The listing builds one solid part. Answer for the finished solid, in the listing's coordinates (mm). Give positions to 0.01 mm unless a question says otherwise; leave off trailing zeros. Order: outer loops, then holes, each group sorted by start corner. A loop starts at its lowest first (then second) coordinate and runs counter-clockwise, first axis right, second up. Notation, with made-up numbers: (21.5, 89.5) - (62.5, 89.5) arc R25 ccw to (62.5, 106.5) - close; hole circle Ø3 at (-22, 60.5). An arc over 180 degrees is marked (long way). Answer in a Markdown table with one row per item. Add a question column.
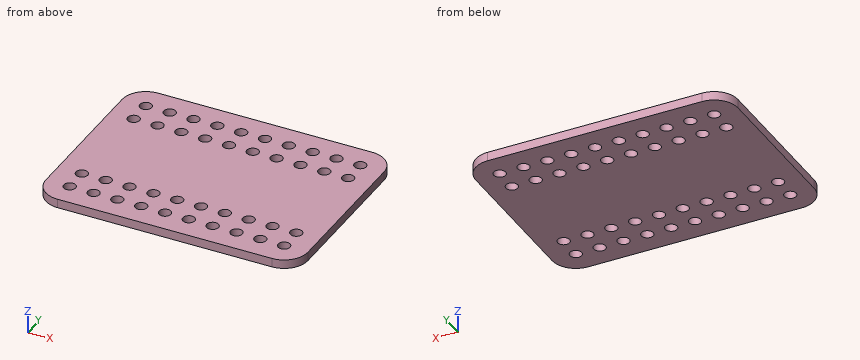
Autodesk Inventor part; units mm, degrees
ref_plane "YZ Plane" through (0, 0, 0) normal (1, 0, 0) x (0, 1, 0)
ref_plane "XZ Plane" through (0, 0, 0) normal (0, 1, 0) x (-1, 0, 0)
ref_plane "XY Plane" through (0, 0, 0) normal (0, 0, 1) x (1, 0, 0)
sketch "Sketch1" plane through (0, 0, 0) normal (0, 0, 1) x (1, 0, 0)
  line L0 (0, 0) -> (558.8, 0)
  line L1 (558.8, 0) -> (558.8, 419.1)
  line L2 (558.8, 419.1) -> (0, 419.1)
  line L3 (0, 419.1) -> (0, 0)
  dimension "d0" = 558.8
  dimension "d1" = 419.1
extrude "Extrusion1" add sketch "Sketch1" along normal blind 19.05
fillet "Fillet1" radius 50.8 1 edges at (558.8, 419.1, 9.525)
fillet "Fillet2" radius 50.8 1 edges at (558.8, 0, 9.525)
fillet "Fillet3" radius 50.8 1 edges at (0, 419.1, 9.525)
fillet "Fillet4" radius 50.8 1 edges at (0, 0, 9.525)
sketch "Sketch2" plane through (0, 0, 19.05) normal (0, 0, 1) x (1, 0, 0)
  arc A0 (558.8, 368.3) -> (508, 419.1) centre (508, 368.3) ccw
  line L0 (0, 368.3) -> (0, 50.8)
  circle A1 centre (50.8, 368.3) radius 12.7
  line L1 (50.8, 368.3) -> (101.6, 368.3)
  line L2 (101.6, 368.3) -> (101.6, 317.5)
  line L3 (50.8, 368.3) -> (50.8, 317.5)
  line L4 (101.6, 368.3) -> (152.4, 368.3)
  line L5 (152.4, 368.3) -> (203.2, 368.3)
  line L6 (203.2, 368.3) -> (254, 368.3)
  line L7 (254, 368.3) -> (304.8, 368.3)
  line L8 (304.8, 368.3) -> (355.6, 368.3)
  line L9 (355.6, 368.3) -> (406.4, 368.3)
  line L10 (406.4, 368.3) -> (457.2, 368.3)
  line L11 (457.2, 368.3) -> (508, 368.3)
  line L12 (508, 368.3) -> (508, 317.5)
  line L13 (457.2, 368.3) -> (457.2, 317.5)
  line L14 (406.4, 368.3) -> (406.4, 317.5)
  line L15 (355.6, 368.3) -> (355.6, 317.5)
  line L16 (304.8, 368.3) -> (304.8, 317.5)
  line L17 (254, 368.3) -> (254, 317.5)
  line L18 (203.2, 368.3) -> (203.2, 317.5)
  line L19 (152.4, 368.3) -> (152.4, 317.5)
  circle A2 centre (101.6, 368.3) radius 12.7
  circle A3 centre (152.4, 368.3) radius 12.7
  circle A4 centre (203.2, 368.3) radius 12.7
  circle A5 centre (254, 368.3) radius 12.7
  circle A6 centre (304.8, 368.3) radius 12.7
  circle A7 centre (355.6, 368.3) radius 12.7
  circle A8 centre (406.4, 368.3) radius 12.7
  circle A9 centre (457.2, 368.3) radius 12.7
  circle A10 centre (508, 368.3) radius 12.7
  circle A11 centre (508, 317.5) radius 12.7
  circle A12 centre (457.2, 317.5) radius 12.7
  circle A13 centre (406.4, 317.5) radius 12.7
  circle A14 centre (355.6, 317.5) radius 12.7
  circle A15 centre (304.8, 317.5) radius 12.7
  circle A16 centre (254, 317.5) radius 12.7
  circle A17 centre (203.2, 317.5) radius 12.7
  circle A18 centre (152.4, 317.5) radius 12.7
  circle A19 centre (101.6, 317.5) radius 12.7
  circle A20 centre (50.8, 317.5) radius 12.7
  circle A21 centre (50.8, 101.6) radius 12.7
  line L20 (50.8, 101.6) -> (101.6, 101.6)
  line L21 (101.6, 101.6) -> (101.6, 50.8)
  line L22 (50.8, 101.6) -> (50.8, 50.8)
  line L23 (101.6, 101.6) -> (152.4, 101.6)
  line L24 (152.4, 101.6) -> (203.2, 101.6)
  line L25 (203.2, 101.6) -> (254, 101.6)
  line L26 (254, 101.6) -> (304.8, 101.6)
  line L27 (304.8, 101.6) -> (355.6, 101.6)
  line L28 (355.6, 101.6) -> (406.4, 101.6)
  line L29 (406.4, 101.6) -> (457.2, 101.6)
  line L30 (457.2, 101.6) -> (508, 101.6)
  line L31 (508, 101.6) -> (508, 50.8)
  line L32 (457.2, 101.6) -> (457.2, 50.8)
  line L33 (406.4, 101.6) -> (406.4, 50.8)
  line L34 (355.6, 101.6) -> (355.6, 50.8)
  line L35 (304.8, 101.6) -> (304.8, 50.8)
  line L36 (254, 101.6) -> (254, 50.8)
  line L37 (203.2, 101.6) -> (203.2, 50.8)
  line L38 (152.4, 101.6) -> (152.4, 50.8)
  circle A22 centre (101.6, 101.6) radius 12.7
  circle A23 centre (152.4, 101.6) radius 12.7
  circle A24 centre (203.2, 101.6) radius 12.7
  circle A25 centre (254, 101.6) radius 12.7
  circle A26 centre (304.8, 101.6) radius 12.7
  circle A27 centre (355.6, 101.6) radius 12.7
  circle A28 centre (406.4, 101.6) radius 12.7
  circle A29 centre (457.2, 101.6) radius 12.7
  circle A30 centre (508, 101.6) radius 12.7
  circle A31 centre (508, 50.8) radius 12.7
  circle A32 centre (457.2, 50.8) radius 12.7
  circle A33 centre (406.4, 50.8) radius 12.7
  circle A34 centre (355.6, 50.8) radius 12.7
  circle A35 centre (304.8, 50.8) radius 12.7
  circle A36 centre (254, 50.8) radius 12.7
  circle A37 centre (203.2, 50.8) radius 12.7
  circle A38 centre (152.4, 50.8) radius 12.7
  circle A39 centre (101.6, 50.8) radius 12.7
  circle A40 centre (50.8, 50.8) radius 12.7
  point P0 (0, 0)
  dimension "d8" = 25.4
  dimension "d9" = 50.8
  dimension "d10" = 50.8
  dimension "d11" = 50.8
  dimension "d12" = 50.8
  dimension "d13" = 50.8
  dimension "d14" = 50.8
  dimension "d15" = 50.8
  dimension "d16" = 50.8
  dimension "d17" = 50.8
  dimension "d18" = 50.8
  dimension "d19" = 50.8
  dimension "d20" = 50.8
  dimension "d21" = 50.8
  dimension "d22" = 50.8
  dimension "d23" = 50.8
  dimension "d24" = 50.8
  dimension "d25" = 50.8
  dimension "d26" = 50.8
  dimension "d27" = 50.8
  dimension "d28" = 25.4
  dimension "d29" = 25.4
  dimension "d30" = 25.4
  dimension "d31" = 25.4
  dimension "d32" = 25.4
  dimension "d33" = 25.4
  dimension "d34" = 25.4
  dimension "d35" = 25.4
  dimension "d36" = 25.4
  dimension "d37" = 25.4
  dimension "d38" = 25.4
  dimension "d39" = 25.4
  dimension "d40" = 25.4
  dimension "d41" = 25.4
  dimension "d42" = 25.4
  dimension "d43" = 25.4
  dimension "d44" = 25.4
  dimension "d45" = 25.4
  dimension "d46" = 25.4
  dimension "d47" = 25.4
  dimension "d48" = 50.8
  dimension "d49" = 50.8
  dimension "d50" = 50.8
  dimension "d51" = 50.8
  dimension "d52" = 50.8
  dimension "d53" = 50.8
  dimension "d54" = 50.8
  dimension "d55" = 50.8
  dimension "d56" = 50.8
  dimension "d57" = 50.8
  dimension "d58" = 50.8
  dimension "d59" = 50.8
  dimension "d60" = 50.8
  dimension "d61" = 50.8
  dimension "d62" = 50.8
  dimension "d63" = 50.8
  dimension "d64" = 50.8
  dimension "d65" = 50.8
  dimension "d66" = 50.8
  dimension "d67" = 25.4
  dimension "d68" = 25.4
  dimension "d69" = 25.4
  dimension "d70" = 25.4
  dimension "d71" = 25.4
extrude "Extrusion2" cut sketch "Sketch2" against normal blind 19.05
properties part number "ROV-Bottom Panel" material "Acetal Resin, Black"
(1) This flat-tipped pin is pushed along its axis until it touches: P1, Ø2, axis at x = 77, y = 279.5, coming from the -Z side. Where does it stop, or does it pass through?
(2) Straight lines are drawn through the part: line 1 (Y direction, x = 203.2, z = 6.5); line 2 (Y direction, x = 363, z = 14.75); line 3 (X direction, y = 399, z = 6.25). For each, find the intervals that lie inside material, in ascending order.
(3) Find section A-A, the plane x = 304.8. Write down the section's boundary in (y, z).
(4) Find section D-D, the plane y = 393.5. Write down the section's boundary in (x, z), plus the area to 3 significant figures.
(5) Find section B-B, the plane y = 101.6. Give the number of separate pieces and of enclosed holes in the cut face, plus the area to 3 significant figures.
Answer key:
| question | item | result |
|---|---|---|
| 1 | P1 | z = 0 |
| 2 | line 1 | 0 to 38.1, 63.5 to 88.9, 114.3 to 304.8, 330.2 to 355.6, 381 to 419.1 |
| 2 | line 2 | 0 to 40.48, 61.12 to 91.28, 111.92 to 307.18, 327.82 to 357.98, 378.62 to 419.1 |
| 2 | line 3 | 10.33 to 548.47 |
| 3 | outline | (0, 0) - (38.1, 0) - (38.1, 19.05) - (0, 19.05) - close; (63.5, 0) - (88.9, 0) - (88.9, 19.05) - (63.5, 19.05) - close; (114.3, 0) - (304.8, 0) - (304.8, 19.05) - (114.3, 19.05) - close; (330.2, 0) - (355.6, 0) - (355.6, 19.05) - (330.2, 19.05) - close; (381, 0) - (419.1, 0) - (419.1, 19.05) - (381, 19.05) - close |
| 4 | outline | (6.69, 0) - (552.11, 0) - (552.11, 19.05) - (6.69, 19.05) - close |
| 4 | area | 10,400 mm² |
| 5 | separate pieces | 11 |
| 5 | enclosed holes | 0 |
| 5 | area | 5,810 mm² |
